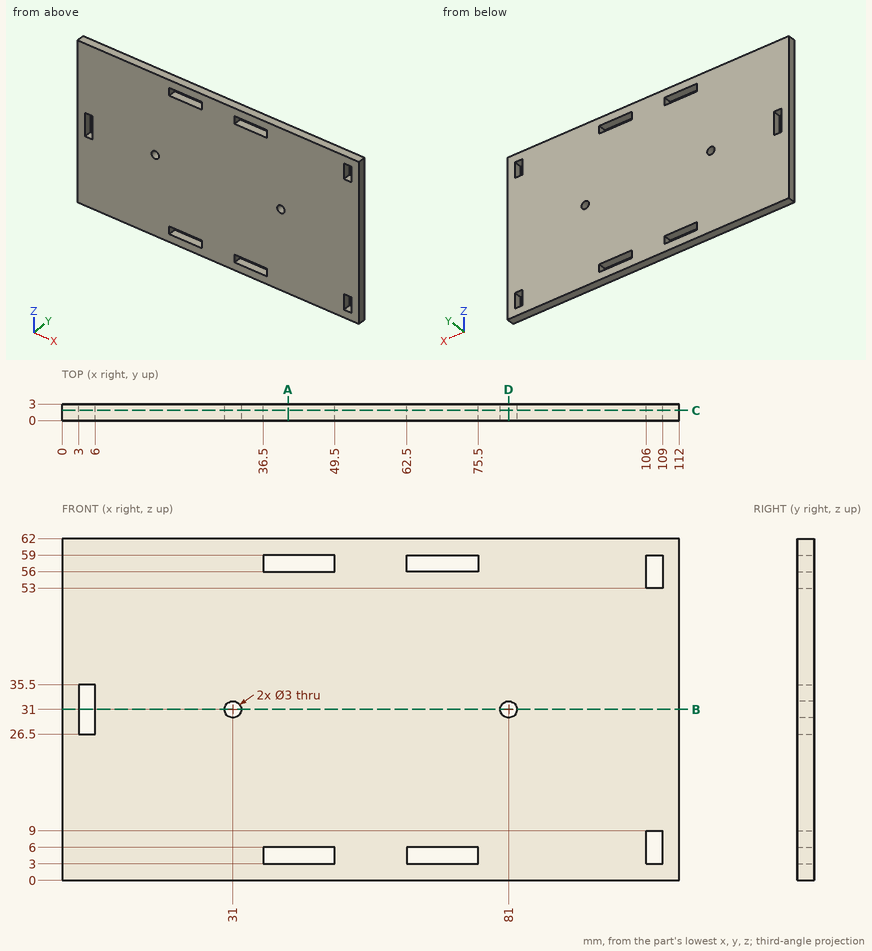
Geometry check sheet. Reference: drawing and pictorial views, mm from the part's lowest x, y, z. Give positions to 0.01 mm unless a question says otherwise; leave off trailing zeros. Order: outer loops, then holes, each group sorted by start corner. A loop starts at its lowest first (then second) coordinate and runs counter-clockwise, first axis right, second up. Notation, with made-up numbers: M 51.25,10.25 L 63.25,10.25 A30 cw 63.25,41.25 Z; hole C 84,85.5 d2. An arc over 180 degrees is marked long. Answer as CSV lines item,"result". Start each with the question number.
Item 1: Cross-section at A-A on x = 41. Enter the section's corners in (y, z), plus the area to 3 significant figures.
Item 2: Cross-section at D-D on x = 81. Enter the section's corners in (y, z).
Item 3: Thickness scan on line 1 (Z direction, x = 46, y = 0.55); line 2 (X direction, y = 0.7, z = 58); line 3 (Z direction, x = 81, y = 2.25). Record the ranges inside material, lowest first. Write a range as [from, to].
Item 4: Cross-section at B-B on z = 31. Enter the section's corners in (x, y).
Item 5: Cross-section at C-C on y = 1.85. State how many separate pieces and enclosed holes the cut face has, plus the area to 3 significant figures.
Established:
1,outline,"M 0,0 L 3,0 L 3,3 L 0,3 Z; M 0,6 L 3,6 L 3,56 L 0,56 Z; M 0,59 L 3,59 L 3,62 L 0,62 Z"
1,area,"168 mm^2"
2,outline,"M 0,0 L 3,0 L 3,29.5 L 0,29.5 Z; M 0,32.5 L 3,32.5 L 3,62 L 0,62 Z"
3,line 1,"z = [0, 3], [6, 56], [59, 62]"
3,line 2,"x = [0, 36.5], [49.5, 62.5], [75.5, 106], [109, 112]"
3,line 3,"z = [0, 29.5], [32.5, 62]"
4,outline,"M 0,0 L 3,0 L 3,3 L 0,3 Z; M 6,0 L 29.5,0 L 29.5,3 L 6,3 Z; M 32.5,0 L 79.5,0 L 79.5,3 L 32.5,3 Z; M 82.5,0 L 112,0 L 112,3 L 82.5,3 Z"
5,separate pieces,"1"
5,enclosed holes,"9"
5,area,"6,710 mm^2"
